Print and shaded views of the part. All mm, measured from the part's lowest x, y and z. Round coordinates to 2 decimals unless told otherwise and drop trailing zeros. Loops run counter-clockwise (first coordinate to the right, second up) from the corner with the lowest first, then second, coordinate; pieces in that order, holes last. Notation, with made-up numbers: (85.5, -21) - (105.5, -21) arc R20 cw to (105.5, -3) - close; hole circle Ø1 at (43.25, -34.75). An arc over 180 degrees is marked (long way). Use one line per item in the form item = value.
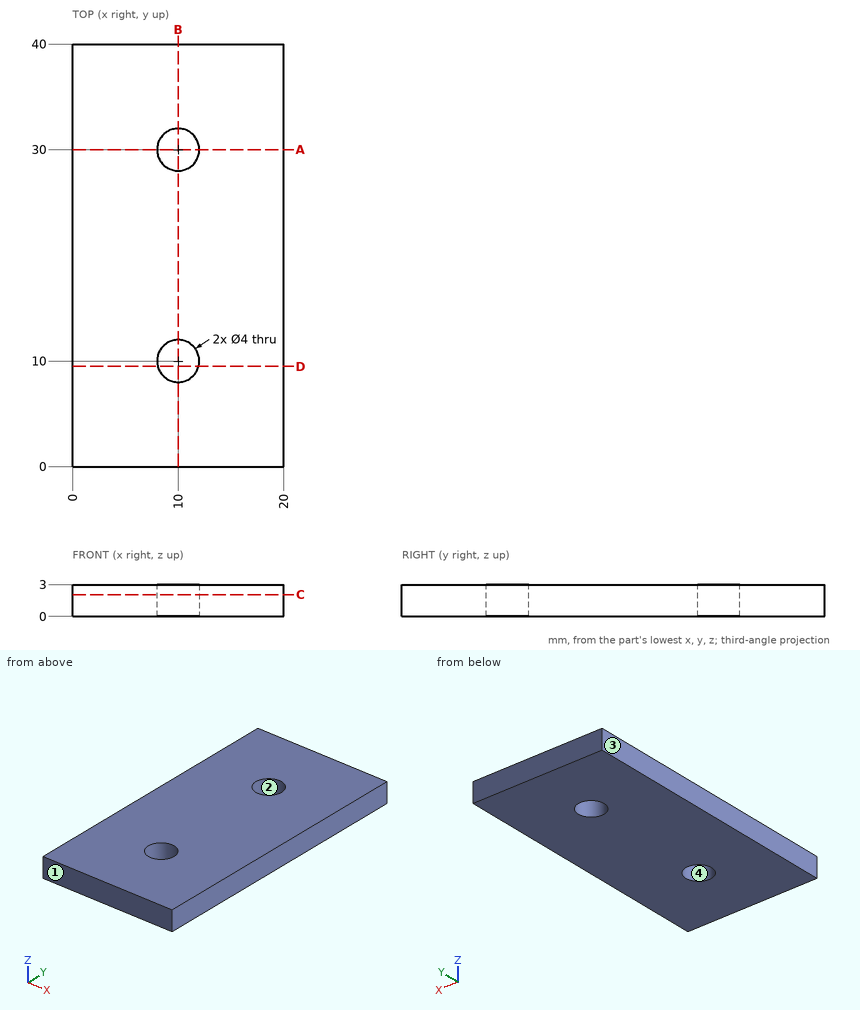
1) Flat gauge pin, fed straight in: pin 1 (5 mm diameter, centred on x = 16, y = 35, fed in from -Z). Where does the tip first touch, or does it go through?
Report:
pin_1 = 0
2) Slice it at D-D (y = 9.5). Write the cut outline in (x, z).
Report:
outline = (0, 0) - (8.06, 0) - (8.06, 3) - (0, 3) - close; (11.94, 0) - (20, 0) - (20, 3) - (11.94, 3) - close
3) Drill centre lines: probe 1 along Y at (x, z) = (10, 0.6); probe 2 along Y at (x, z) = (9.5, 1.85). Where is each one in solid material? Low to high.
Report:
probe_1 = 0 to 8, 12 to 28, 32 to 40
probe_2 = 0 to 8.06, 11.94 to 28.06, 31.94 to 40
4) Slice it at B-B (x = 10). Write the cut outline in (y, z), plus the area to 3 significant figures.
Report:
outline = (0, 0) - (8, 0) - (8, 3) - (0, 3) - close; (12, 0) - (28, 0) - (28, 3) - (12, 3) - close; (32, 0) - (40, 0) - (40, 3) - (32, 3) - close
area = 96.0 mm^2
5) Slice it at A-A (y = 30). Write the cut outline in (x, z), plus the area to 3 significant figures.
Report:
outline = (0, 0) - (8, 0) - (8, 3) - (0, 3) - close; (12, 0) - (20, 0) - (20, 3) - (12, 3) - close
area = 48.0 mm^2
6) Slice it at C-C (z = 2.05). Write the cut outline in (x, y).
Report:
outline = (0, 0) - (20, 0) - (20, 40) - (0, 40) - close; hole circle Ø4 at (10, 10); hole circle Ø4 at (10, 30)
7) Two-plate mould, pull along X, no slides. Class the marked faces 1, 2, 3 and 4: +X half, -X half, draft (parallel to the pull), parting line (faces both ways), or undercut.
Report:
face_1 = draft
face_2 = undercut
face_3 = -X half
face_4 = undercut
